The model under review builds one solid part; all positions refer to its coordinate system, in mm. Face numbers are marked on the shaded views. A direction names the side the tool comes from. Round coordinates to 2 decimals unless told otherwise and drop trailing zeros. Order: outer loops, then holes, each group sorted by start corner. A loop starts at its lowest first (then second) coordinate and runs counter-clockwise, first axis right, second up. Notation, with made-up numbers: (-26.5, 83) -> (-2.5, 83) arc R28 ccw to (-2.5, 109) -> close; hole circle Ø5 at (-24, -20.5). An arc over 180 degrees is marked (long way). Use a Markdown table: item, result. Add a question column.
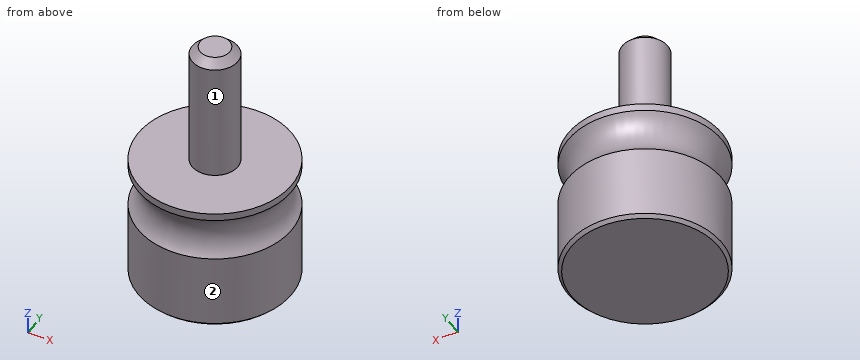
```python
from build123d import *

# Parameters (mm, degrees)
SKETCH1_R           = 4.7625
BOSS_EXTRUDE1_DEPTH = 4.7625
SKETCH3_R           = 1.4224
BOSS_EXTRUDE2_DEPTH = 7.9375
CHAMFER1_SIZE       = 0.2
CHAMFER2_SIZE       = 0.5


with BuildPart() as part:
    # Sketch1 → Boss-Extrude1 (new body)
    with BuildSketch(Plane.XY):
        with Locations(Location((0, 0, 0), (0, 0, 180))):
            Circle(SKETCH1_R)
    extrude(amount=BOSS_EXTRUDE1_DEPTH)

    # Sketch2 → Revolve1 (revolve)
    with BuildSketch(Plane(origin=(0, 0, 0), x_dir=(1, 0, 0), z_dir=(0, 1, 0)), mode=Mode.PRIVATE) as revolve1_sk:
        with BuildLine():
            Line((-4.7625, -7.477150663), (-4.7625, -7.9375))
            Line((-4.7625, -7.9375), (0, -7.9375))
            Line((0, -7.9375), (0, -4.7625))
            Line((0, -4.7625), (-4.7625, -4.7625))
            ThreePointArc((-4.7625, -4.7625), (-4.200277439, -6.119825331), (-4.7625, -7.477150663))
        make_face()
    revolve(revolve1_sk.sketch.rotate(Axis((0, 0, 7.9375), (0, 0, -1)), 180), axis=Axis((0, 0, 7.9375), (0, 0, -1)))

    # Sketch3 → Boss-Extrude2 (add)
    with BuildSketch(Plane.XY.offset(7.9375)):
        with Locations(Location((0, 0, 0), (0, 0, 180))):
            Circle(SKETCH3_R)
    extrude(amount=BOSS_EXTRUDE2_DEPTH)

    # Chamfer1
    chamfer1_edges = [part.edges().sort_by_distance(p)[0] for p in [
        (4.7625, 0, 0),
    ]]
    chamfer(chamfer1_edges, length=CHAMFER1_SIZE)

    # Chamfer2
    chamfer2_edges = [part.edges().sort_by_distance(p)[0] for p in [
        (1.4224, 0, 15.875),
    ]]
    chamfer(chamfer2_edges, length=CHAMFER2_SIZE)


solid = part.part
```
Q1. Add section C-C, the plane z = 4. Give the boundary of the cut face in (x, y) (1 decimal).
Q2. For the marked faces 1 and 2, list the 3-axis set-ups (+Z, -Z, +X, -X, +Y, -Y) from which the entire face can be reached by the end or side of a thin tool; tool diameter is ignored.
Q3. Add section D-D, the plane z = 13.25. Give the boundary of the cut face in (x, y).
Q4. For pin 1 (1 mm diameter, centred on x = 2.5, z = 1.5, fed in from +Y); pin 2 (5 mm diameter, centred on x = -3, z = 14, fed in from +Y); pin 3 (3 mm diameter, centred on x = -2.5, y = 3, fed in from -Z), all flat-tipped, find the tip position at first contact; note any pin that passes through.
Q5. To check wall thickness, follow line 1 along Z through (x, y) = (1.5, 2.5); line 2 along Y through (x, z) = (-2.25, 5.75); line 3 along X through (y, z) = (0.25, 3.5). State the ranges of each line that lie inside material, in increasing order.
Return value:
| question | item | result |
|---|---|---|
| 1 | outline | circle Ø9.5 at (0, 0) |
| 2 | face 1 | +Z |
| 2 | face 2 | +Z, -Z |
| 3 | outline | circle Ø2.84 at (0, 0) |
| 4 | pin 1 | y = 4.32 |
| 4 | pin 2 | y = 1.33 |
| 4 | pin 3 | z = 0 |
| 5 | line 1 | 0 to 7.94 |
| 5 | line 2 | -3.59 to 3.59 |
| 5 | line 3 | -4.76 to 4.76 |
